from build123d import *

# Parameters (mm, degrees)
F2_R     = 1
F3_DEPTH = 12.5


with BuildPart() as f1:
    # F0 (on Front) → F1 (revolve)
    with BuildSketch(Plane.XZ):
        with BuildLine():
            Line((-31.7, 2.5), (-45, 2.5))
            Line((-45, 2.5), (-45, 0))
            Line((-45, 0), (45, 0))
            Line((45, 0), (45, 2.5))
            Line((45, 2.5), (31.7, 2.5))
            Line((31.7, 2.5), (31.7, 2.2))
            ThreePointArc((31.7, 2.2), (31.641421, 2.058579), (31.5, 2))
            Line((31.5, 2), (31.2, 2))
            ThreePointArc((31.2, 2), (31.058579, 2.058579), (31, 2.2))
            Line((31, 2.2), (31, 2.5))
            Line((31, 2.5), (-31, 2.5))
            Line((-31, 2.5), (-31, 2.2))
            ThreePointArc((-31, 2.2), (-31.058579, 2.058579), (-31.2, 2))
            Line((-31.2, 2), (-31.5, 2))
            ThreePointArc((-31.5, 2), (-31.641421, 2.058579), (-31.7, 2.2))
            Line((-31.7, 2.2), (-31.7, 2.5))
        make_face()
    revolve(axis=Axis((0, 0, 0), (1, 0, 0)))

    # F2 (on Top) → F3 (cut, symmetric)
    with BuildSketch(Plane.XY):
        with Locations((-43, 0)):
            Circle(F2_R)
        Circle(F2_R)
        with Locations((43, 0)):
            Circle(F2_R)
    extrude(amount=F3_DEPTH, both=True, mode=Mode.SUBTRACT)


solid = f1.part
Can you work these out from the model? Positions are in its coordinate system, mm. Round coordinates to 2 decimals unless told otherwise and drop trailing zeros. Order: outer loops, then holes, each group sorted by start corner. A loop starts at its lowest first (then second) coordinate and runs counter-clockwise, first axis right, second up. Notation, with made-up numbers: (70, 25) - (119, 25) arc R22 ccw to (119, 50) - close; hole circle Ø9 at (-25, -6). An arc over 180 degrees is marked (long way). Answer in a Markdown table with one row per item.
(1) Please list where these lines run through material, in increasing order: L1, parallel to X at y = 0, z = 0.8; L2, parallel to X at y = -2.3, z = -0.2; L3, parallel to Y at x = 0, z = 1.5. Write a range as from..to.
From the geometry:
| item | result |
|---|---|
| L1 | x = -45..-44, -42..-1, 1..42, 44..45 |
| L2 | x = -45..-31.7, -31..31, 31.7..45 |
| L3 | y = -2..-1, 1..2 |
(2) If we mould it in two halves opening along Y, with no side actions, what happens to faces 1 (the face through (-38.4, -0.1, -2.5)), 2 (the face through (44, 0, 0)), 3 (the face through (-45, 0, 0))? For each: released by +Y, released by -Y, zero draft, split by the parting line, or undercut.
From the geometry:
| item | result |
|---|---|
| face 1 | split by the parting line |
| face 2 | undercut |
| face 3 | zero draft |
(3) Suppose I cut it at C-C, the plane x = -33. Please give me the cut outline in (y, z).
From the geometry:
| item | result |
|---|---|
| outline | circle Ø5 at (0, 0) |
(4) For P1, Ø2.5, axis at x = 43, y = 0, coming from the +Z side, with a flat end and sliding along its axis, tell me the tip position at first contact or that it passes through.
From the geometry:
| item | result |
|---|---|
| P1 | stops at z = 2.5 |
(5) Suppose I cut it at A-A, the plane y = 0. Count the separate pieces of the cut face and the enclosed holes in it, plus the area to 3 significant figures.
From the geometry:
| item | result |
|---|---|
| separate pieces | 4 |
| enclosed holes | 0 |
| area | 419 mm2 |
(6) Suppose I cut it at B-B, the plane x = -43. Please give me the cut outline in (y, z).
From the geometry:
| item | result |
|---|---|
| outline | (-1, -2.29) - (-1, 2.29) arc R2.5 ccw to start; (1, -2.29) arc R2.5 ccw to (1, 2.29) - close |
